The figure shows three views and two pictorial views of one solid part (mm, origin at its lowest corner). Answer the questions. A direction names the side the tool comes from. Round coordinates to 2 decimals unless told otherwise and drop trailing zeros. Write each loop counter-clockwise with the first axis right and the second up, starting at its lowest first coordinate (ties: lowest second). Pieces come first, ordered by that corner, then holes. Notation, with made-up numbers: M -39,82 L 10,82 A17 ccw 10,103 Z; hole C -33.75,-24.5 d11. An arc over 180 degrees is marked long. Use one line per item in the form item = value. Start each with the question number.
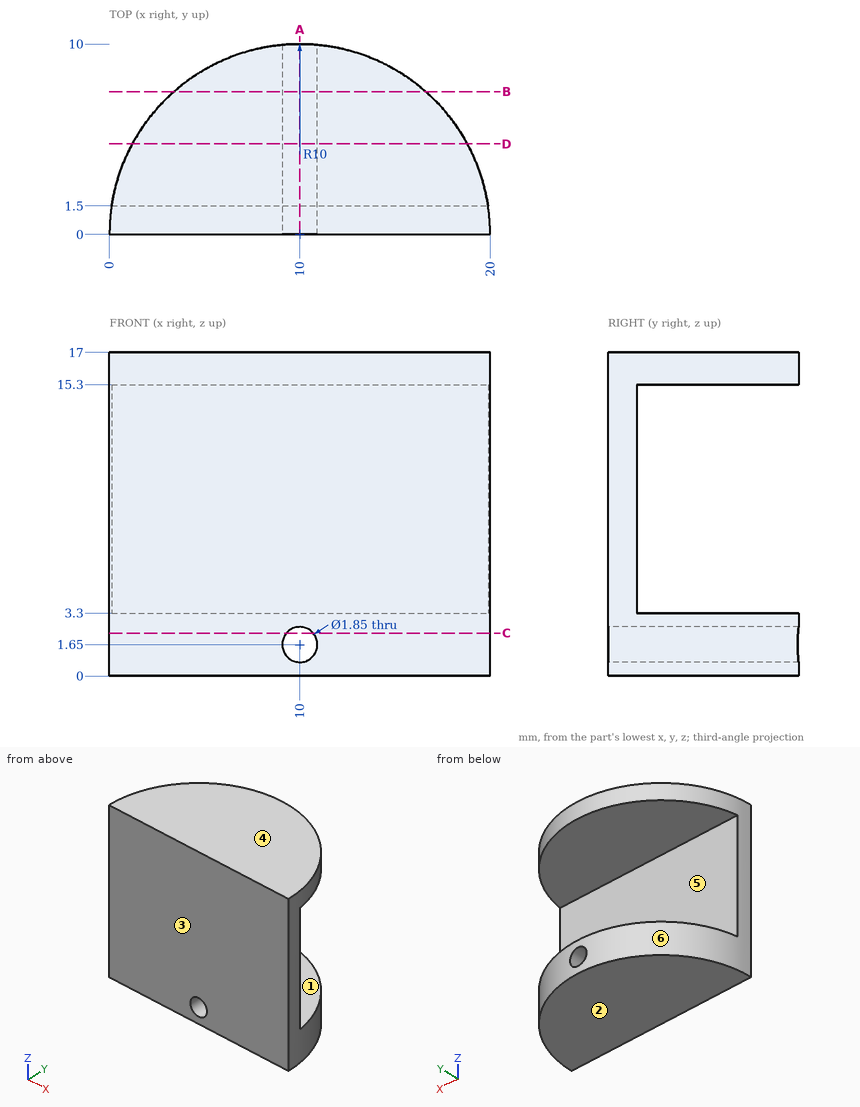
Q1. Find section C-C on z = 2.25. Write down the section's boundary in (x, y), and give its area (3 significant figures).
Q2. Each of these flat-tipped pins is pushed along its axis until it touches: pin 1 Ø5 at (x, z) = (17, 9.5) entering from +Y; pin 2 Ø10 at (x, z) = (17, 6) entering from +Y. Where does it stop, or does it pass through?
Q3. Find section B-B on y = 7.5. Write down the section's boundary in (x, z) (3 decimals), and give its area (3 significant figures).
Q4. Straight lines are drawn through the part: line 1 (Z direction, x = 10, y = 3.5) (3 decimals); line 2 (Z direction, x = 16.25, y = 5.25); line 3 (Y direction, x = 15.5, z = 5.25). For each, find the intervals that lie inside material, in ascending order. Write a range as [from, to].
Q5. For a pull along Z with two mould halves and no side action, classify the marked faces 1, 2, 3 and 4 as +Z half, -Z half, draft (parallel to the pull), parting line (faces both ways), or undercut.
Q6. A tool of negligible diameter and unlimited length cuts with its end or side. For the marked faces 5 and 6, from which of +Z, -Z, +X, -X, +Y, -Y can it reach the whole face along a straight path? Write none if from no direction.
Q7. Find section D-D on y = 4.75. Write down the section's boundary in (x, z) (3 decimals).
Q8. Find section A-A on x = 10. Write down the section's boundary in (y, z) (3 decimals), and give its area (3 significant figures).
Response:
q1.outline = M 0,0 L 9.3,0 L 9.3,9.98 A10 ccw Z; M 10.7,0 L 20,0 A10 ccw 10.7,9.98 Z
q1.area = 143 mm²
q2.pin_1 = 1.5
q2.pin_2 = 9.6
q3.outline = M 3.386,0 L 16.614,0 L 16.614,3.3 L 3.386,3.3 Z; M 3.386,15.3 L 16.614,15.3 L 16.614,17 L 3.386,17 Z; hole C 10,1.65 d1.85
q3.area = 63.5 mm²
q4.line_1 = [0, 0.725], [2.575, 3.3], [15.3, 17]
q4.line_2 = [0, 3.3], [15.3, 17]
q4.line_3 = [0, 1.5]
q5.face_1 = undercut
q5.face_2 = -Z half
q5.face_3 = draft
q5.face_4 = +Z half
q6.face_5 = +X, -X, +Y
q6.face_6 = +Z, -Z, +Y
q7.outline = M 1.2,0 L 18.8,0 L 18.8,3.3 L 1.2,3.3 Z; M 1.2,15.3 L 18.8,15.3 L 18.8,17 L 1.2,17 Z; hole C 10,1.65 d1.85
q8.outline = M 0,0 L 10,0 L 10,0.725 L 0,0.725 Z; M 0,2.575 L 10,2.575 L 10,3.3 L 1.5,3.3 L 1.5,15.3 L 10,15.3 L 10,17 L 0,17 Z
q8.area = 49.5 mm²
